from build123d import *

# Parameters (mm, degrees)
SKETCH2_R          = 6.35
CUT_EXTRUDE1_DEPTH = 76.201267443
CIRPATTERN1_COUNT  = 6


with BuildPart() as part:
    # Sketch1 → Revolve1 (revolve)
    with BuildSketch(Plane.XY, mode=Mode.PRIVATE) as revolve1_sk:
        Polygon((0, 50.8), (0, 9.525), (19.05, 9.525), (19.05, 15.875), (3.175, 19.05), (3.175, 44.45), (12.7, 47.625), (12.7, 50.8), align=None)
    revolve1 = revolve(revolve1_sk.sketch.rotate(Axis((0, 0, 0), (1, 0, 0)), 90), axis=Axis((0, 0, 0), (1, 0, 0)))

    # Mirror1: Revolve1 across plane
    add(revolve1.mirror(Plane(origin=(0, 50.8, 0), x_dir=(0, 0, 1), z_dir=(1, 0, 0))))

    # Sketch2 → Cut-Extrude1 (cut, through all)
    with BuildSketch(Plane(origin=(3.175, 0, 0), x_dir=(0, 0, -1), z_dir=(1, 0, 0))):
        with Locations((27.49630657, 15.875)):
            Circle(SKETCH2_R)
    cut_extrude1 = extrude(amount=-CUT_EXTRUDE1_DEPTH, mode=Mode.SUBTRACT)

    # CirPattern1: Cut-Extrude1 ×6 about axis
    cirpattern1_axis = Axis((0, 0, 0), (1, 0, 0))
    for i in range(1, CIRPATTERN1_COUNT):
        add(cut_extrude1.rotate(cirpattern1_axis, i * 360 / CIRPATTERN1_COUNT), mode=Mode.SUBTRACT)


solid = part.part
Read the model definition and answer for the solid it produces. Units are mm, in the model's axes. A direction names the side the tool comes from. Round coordinates to 2 decimals unless told otherwise and drop trailing zeros. Write each loop counter-clockwise with the first axis right and the second up, starting at its lowest first coordinate (ties: lowest second). Pieces come first, ordered by that corner, then holes.
1. The part is cut by section B-B, the plane y = 0. Determine the outline of the cut face in (x, z) (3 decimals).
2. Given pin 1 Ø1 at (x, y) = (13.5, 33.5) entering from -Z; pin 2 Ø20.5 at (y, z) = (15.87, 27.5) entering from -X (3 decimals); pin 3 Ø5 at (y, z) = (16.5, 35.5) entering from +X (3 decimals); pin 4 Ø1.5 at (x, z) = (-1, -6.5) entering from -Y, each flat-ended and moving along its own axis, determine where each tip first touches the part or whether it passes through.
3. The part is cut by section D-D, the plane x = -9. Determine the outline of the cut face in (y, z) (3 decimals), then the cut area to 3 significant figures.
4. The part is cut by section A-A, the plane z = 0. State how many separate pieces and enclosed holes the cut face has, then the cut area to 3 significant figures.
5. Straight lines are drawn through the part: L1, parallel to Y at x = -1.25, z = 0 (3 decimals); L2, parallel to Z at x = -4, y = -2.5; L3, parallel to Z at x = -12, y = 12. For each, find the intervals that lie inside material, in ascending order.
6. Which of the six approach directions +Z, -Z, +X, -X, +Y, -Y give full straight-line access (tool end or side, diameter ignored) to faces 3 (the face through (-3.175, 19, -9)), 4 (the face through (3.175, 19, -9)), 5 (the face through (0.044, -10.241, 30.426))?
7. Determine the mould class of faces 1 (the face through (14.53, 16.38, -3.64)), 2 (the face through (-12.7, -45.4, 15.3)) for opening direction Z: pulls with the +Z half, pulls with the -Z half, needs draft (parallel to the pull), parting line crosses it, or undercut.
8. The part is cut by section C-C, the plane x = 6. Determine the outline of the cut face in (y, z) (3 decimals).
Values:
1. outline: (-19.05, -15.875) - (-3.175, -19.05) - (-3.175, -44.45) - (-12.7, -47.625) - (-12.7, -50.8) - (12.7, -50.8) - (12.7, -47.625) - (3.175, -44.45) - (3.175, -19.05) - (19.05, -15.875) - (19.05, -9.525) - (-19.05, -9.525) - close; (-19.05, 9.525) - (19.05, 9.525) - (19.05, 15.875) - (3.175, 19.05) - (3.175, 44.45) - (12.7, 47.625) - (12.7, 50.8) - (-12.7, 50.8) - (-12.7, 47.625) - (-3.175, 44.45) - (-3.175, 19.05) - (-19.05, 15.875) - close
2. pin 1: passes through
2. pin 2: stops at x = -3.175
2. pin 3: stops at x = 3.175
2. pin 4: stops at y = -50.47
3. outline: circle Ø101.6 at (0, 0); circle Ø35.77 at (0, 0); hole circle Ø92.783 at (0, 0); hole circle Ø19.05 at (0, 0)
3. area: 2,070 mm2
4. separate pieces: 4
4. enclosed holes: 0
4. area: 1,050 mm2
5. L1: y = -50.8 to -38.1, -25.4 to -9.525, 9.525 to 25.4, 38.1 to 50.8
5. L2: z = -50.74 to -44.66, -18.72 to -9.19, 9.19 to 18.72, 44.66 to 50.74
5. L3: z = -49.36 to -45.85, -12.44 to 12.44, 45.85 to 49.36
6. face 3: -X
6. face 4: +X
6. face 5: +X, -X
7. face 1: undercut
7. face 2: needs draft
8. outline: circle Ø101.6 at (0, 0); circle Ø36.97 at (0, 0); hole circle Ø90.783 at (0, 0); hole circle Ø19.05 at (0, 0)
